Read the model definition and answer for the solid it produces. Units are mm, in the model's axes. Coordinates: 2 decimals unless noted, no trailing zeros. Loops run counter-clockwise (first coordinate to the right, second up) from the corner with the lowest first, then second, coordinate; pieces in that order, holes last. Notation, with made-up numbers: (36.25, 84) - (47.25, 84) arc R15 cw to (47.25, 88) - close; hole circle Ø4 at (5.5, 11.25). An arc over 180 degrees is marked (long way). Use one line per item in the form item = value.
Autodesk Inventor part; units mm, degrees
ref_plane "YZ Plane" through (0, 0, 0) normal (1, 0, 0) x (0, 1, 0)
ref_plane "XZ Plane" through (0, 0, 0) normal (0, 1, 0) x (-1, 0, 0)
ref_plane "XY Plane" through (0, 0, 0) normal (0, 0, 1) x (1, 0, 0)
sketch "Sketch1" plane through (0, 0, 0) normal (0, 1, 0) x (-1, 0, 0)
  circle A0 centre (0, 0) radius 152.4 construction
  circle A1 centre (0, 0) radius 203.2 construction
  line L0 (0, 0) -> (0, -94.5056)
  line L1 (0, 0) -> (255.4804, -255.4804) construction
  circle A2 centre (152.4, 0) radius 3.3782
  circle A3 centre (203.2, 0) radius 3.3782
  circle A4 centre (107.7631, -107.7631) radius 3.3782
  circle A5 centre (143.6841, -143.6841) radius 3.3782
  line L2 (250.9903, -259.9706) -> (8.0112, -16.9915)
  line L3 (143.6841, -152.6644) -> (152.6644, -143.6841)
  line L4 (98.7828, -107.7631) -> (107.7631, -98.7828)
  line L5 (146.05, 6.35) -> (209.55, 6.35)
  line L6 (209.55, 6.35) -> (209.55, -6.35)
  line L7 (146.05, -6.35) -> (146.05, 6.35)
  line L8 (152.6644, -143.6841) -> (209.55, -6.35)
  line L9 (146.05, -6.35) -> (107.7631, -98.7828)
  circle A6 centre (175.8001, -60.9582) radius 3.3782
  circle A7 centre (157.3663, -122.0546) radius 3.3782
  circle A8 centre (140.6003, -46.378) radius 3.3782
  circle A9 centre (116.2999, -105.0443) radius 3.3782
  dimension "d34" = 304.8
  dimension "d36" = 406.4
  dimension "d38" = 45
  dimension "d40" = 6.7564
  dimension "d41" = 6.7564
  dimension "d42" = 6.7564
  dimension "d43" = 6.7564
  dimension "d44" = 6.35
  dimension "d45" = 6.35
  dimension "d46" = 6.35
  dimension "d48" = 6.35
  dimension "d49" = 6.35
  dimension "d51" = 6.35
  dimension "d52" = 6.35
  dimension "d53" = 157.5
  dimension "d58" = 6.7564
  dimension "d59" = 6.7564
  dimension "d64" = 6.7564
  dimension "d70" = 6.7564
  dimension "d72" = 63.5
ref_plane "Work Plane1" through (0, 3.175, 0) normal (0, 1, 0) x (1, 0, 0)
extrude "Extrusion5" add sketch "Sketch1" along normal blind 3.175
properties part number "Extender Mounting Plate"
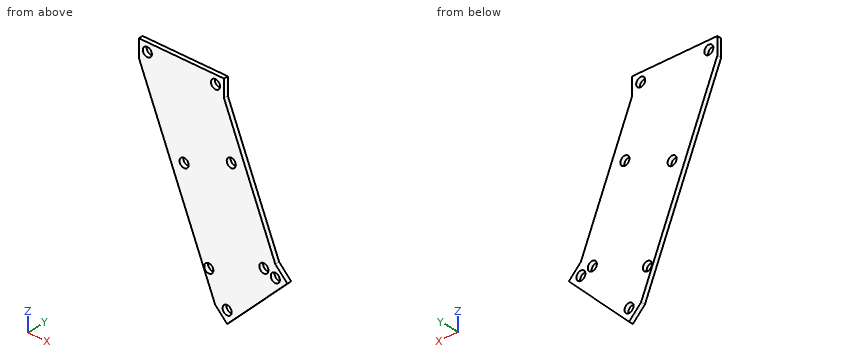
Item 1: The part is cut by section C-C on x = -203.2. Give the vertices of the cut face in (y, z) (3 decimals), plus the area to 3 significant figures.
Results below:
outline = (0, -21.68) - (3.175, -21.68) - (3.175, -3.378) - (0, -3.378) - close; (0, 3.378) - (3.175, 3.378) - (3.175, 6.35) - (0, 6.35) - close
area = 67.5 mm²
Item 2: The part is cut by section B-B on y = 1.45. Count the separate pieces of the cut face and the enclosed holes in it, plus the area to 3 significant figures.
Results below:
separate_pieces = 1
enclosed_holes = 8
area = 8,620 mm²
Item 3: The part is cut by section D-D on z = -133. Give the vertices of the cut face in (x, y) (3 decimals).
Results below:
outline = (-157.09, 0) - (-124.02, 0) - (-124.02, 3.175) - (-157.09, 3.175) - close
Item 4: Each of these flat-tipped pins is pushed along its axis until it touches: P1, Ø6, axis at x = -175.8, z = -60.96, coming from the +Y side; P2, Ø1.5, axis at y = 1, z = -22.5, coming from the +X side. Where does it stop, or does it pass through?
Results below:
P1 = through
P2 = -139.05
Item 5: Find the intervals of material crossed by L1, parallel to X at y = 2.1, z = -142; L2, parallel to Z at x = -105, y = 3.05; L3, parallel to Z at x = -108.5, y = 0.45, in increasing order.
Results below:
L1 = -153.36 to -146.61, -140.76 to -133.02
L2 = -113.98 to -109.71, -105.82 to -101.55
L3 = -117.48 to -111.06, -104.47 to -97
Item 6: The part is cut by section A-A on z = 0. Give the vertices of the cut face in (x, y) (3 decimals).
Results below:
outline = (-209.55, 0) - (-206.578, 0) - (-206.578, 3.175) - (-209.55, 3.175) - close; (-199.822, 0) - (-155.778, 0) - (-155.778, 3.175) - (-199.822, 3.175) - close; (-149.022, 0) - (-146.05, 0) - (-146.05, 3.175) - (-149.022, 3.175) - close
